Build history of the part. All positions in model axes, mm. Face numbers are marked on the shaded views. A direction names the side the tool comes from. Give positions to 0.01 mm unless a question says otherwise; leave off trailing zeros. Write each loop counter-clockwise with the first axis right and the second up, starting at its lowest first coordinate (ties: lowest second). Pieces come first, ordered by that corner, then holes. Notation, with made-up numbers: M 13,-37.5 L 38,-37.5 A21 cw 38,-22.5 Z; hole C 53,59 d1. An arc over 180 degrees is marked long. One line per item, written item: value. Start each with the question number.
from build123d import *

# Parameters (mm, degrees)
SKETCH_1_R          = 20
EXTRUDE_1_DEPTH     = 10
SKETCH_2_R          = 10
CUT_EXTRUDE_1_DEPTH = 5
CUT_EXTRUDE_START   = -5
SKETCH_3_R          = 20
SKETCH_3_R_2        = 15
CUT_EXTRUDE_3_DEPTH = 5
FILLET_1_R          = 2
FILLET_2_R          = 2


with BuildPart() as part:
    # 草图1 → 凸台-拉伸1 (new body)
    with BuildSketch(Plane.XY):
        Circle(SKETCH_1_R)
    extrude(amount=EXTRUDE_1_DEPTH)

    # 草图2 → 切除-拉伸1 (cut)
    with BuildSketch(Plane(origin=(0, 0, 0), x_dir=(-1, 0, 0), z_dir=(0, 0, -1))):
        Circle(SKETCH_2_R)
    extrude(amount=-CUT_EXTRUDE_1_DEPTH, mode=Mode.SUBTRACT)

    # 草图3 → 切除-拉伸3 (cut)
    with BuildSketch(Plane.XY.offset(10).offset(CUT_EXTRUDE_START)):
        Circle(SKETCH_3_R)
        Circle(SKETCH_3_R_2, mode=Mode.SUBTRACT)
    extrude(amount=CUT_EXTRUDE_3_DEPTH, mode=Mode.SUBTRACT)

    # 圆角1
    fillet_1_edges = [part.edges().sort_by_distance(p)[0] for p in [
        (-15, 0, 10),
    ]]
    fillet(fillet_1_edges, radius=FILLET_1_R)

    # 圆角2
    fillet_2_edges = [part.edges().sort_by_distance(p)[0] for p in [
        (-20, 0, 5),
    ]]
    fillet(fillet_2_edges, radius=FILLET_2_R)


solid = part.part
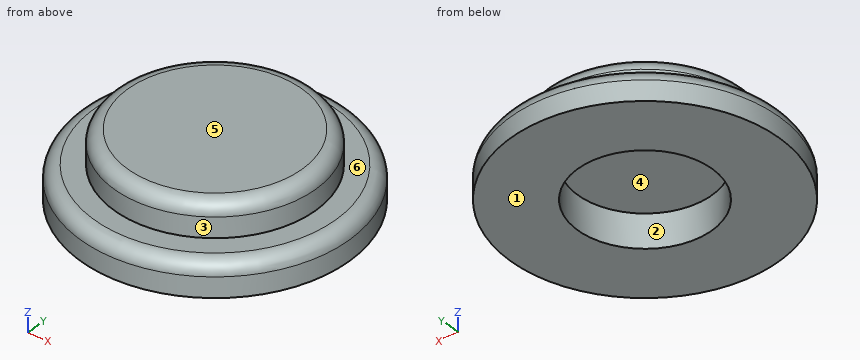
1) Band-saw the part on C-C (z = 2). List the corners of the cut face in (x, y), then the cut area to 3 significant figures.
2) Band-saw the part on D-D (z = 7.5). List the corners of the cut face in (x, y), then the cut area to 3 significant figures.
3) Mould opens along X. For the marked faces 1, 2 and 3 say: released by +X, released by -X, zero draft, split by the parting line, or undercut.
4) Drop flat-ended pins along their axis: P1, Ø1.5, axis at x = 7.5, y = 15, coming from the +Z side; P2, Ø18, axis at x = 0, y = 0, coming from the -Z side; P3, Ø5, axis at x = 5, z = 3.5, coming from the +Y side. Give the stop position or say it passes through.
5) Tool access for the marked faces 4, 5 and 6: list every direction of +Z, -Z, +X, -X, +Y, -Y with a clear straight run to the whole face (end or side of a thin tool).
6) Band-saw the part on A-A (y = 0). List the corners of the cut face in (x, z), then the cut area to 3 significant figures.
7) Probe line 1 along Y through (x, z) = (0, 2.4); line 2 along Z through (x, y) = (10, -15); line 3 along Y through (x, z) = (0.5, 7.25). List the from-to ranges inside material, lowest first. Write a range as from..to.
Model answer:
1. outline: C 0,0 d40; hole C 0,0 d20
1. area: 942 mm²
2. outline: C 0,0 d30
2. area: 707 mm²
3. face 1: zero draft
3. face 2: undercut
3. face 3: split by the parting line
4. P1: stops at z = 5
4. P2: stops at z = 5
4. P3: stops at y = 19.84
5. face 4: -Z
5. face 5: +Z, +X, -X, +Y, -Y
5. face 6: +Z
6. outline: M -20,0 L -10,0 L -10,5 L 10,5 L 10,0 L 20,0 L 20,3 A2 ccw 18,5 L 15,5 L 15,8 A2 ccw 13,10 L -13,10 A2 ccw -15,8 L -15,5 L -18,5 A2 ccw -20,3 Z
6. area: 247 mm²
7. line 1: y = -20..-10, 10..20
7. line 2: z = 0..5
7. line 3: y = -14.99..14.99
